from build123d import *

# Parameters (mm, degrees)
SKETCH2_W               = 42
SKETCH2_H               = 40
BOSS_EXTRUDE1_DEPTH     = 12.15
CUT_EXTRUDE1_DEPTH      = 149.231651478
CUT_EXTRUDE1_DEPTH_BACK = 149.231651478
SKETCH3_R               = 3.25
FILLET1_R               = 25
FILLET2_R               = 5
SKETCH4_R               = 3
BOSS_EXTRUDE2_DEPTH     = 2.8
CHAMFER1_SIZE           = 0.5
SKETCH6_W               = 20
SKETCH6_H               = 10.5
BOSS_EXTRUDE3_DEPTH     = 22
BOSS_EXTRUDE5_DEPTH     = 12
SKETCH7_R               = 1.65
CUT_EXTRUDE2_DEPTH      = 4
FILLET3_R               = 10
CHAMFER3_SIZE           = 2
SKETCH9_R               = 3.25
CUT_EXTRUDE3_DEPTH      = 2


# Some blends are built 0.0001 mm under size
with BuildPart() as part:
    # Sketch2 → Boss-Extrude1 (new, symmetric)
    with BuildSketch(Plane.XY):
        Polygon((-33, 0), (33, 0), (33, -144), (21, -144), (21, -99), (-21, -99), (-21, -144), (-33, -144), align=None)
        with Locations((0, -32)):
            Rectangle(SKETCH2_W, SKETCH2_H, mode=Mode.SUBTRACT)
        with Locations((0, -75.5)):
            Rectangle(SKETCH2_W, SKETCH2_H, mode=Mode.SUBTRACT)
    extrude(amount=BOSS_EXTRUDE1_DEPTH, both=True)

    # Sketch3 → Cut-Extrude1 (cut, two sides: drawn at the far end of the back side and taken through both)
    with BuildSketch(Plane(origin=(0, 0, 0), x_dir=(0, 0, -1), z_dir=(1, 0, 0)).offset(-CUT_EXTRUDE1_DEPTH_BACK)):
        with Locations((0, -106)):
            Circle(SKETCH3_R)
        with Locations((0, -62.5)):
            Circle(SKETCH3_R)
        with Locations((0, -19)):
            Circle(SKETCH3_R)
        with Locations((6, -134)):
            Circle(SKETCH3_R)
    extrude(amount=CUT_EXTRUDE1_DEPTH + CUT_EXTRUDE1_DEPTH_BACK, mode=Mode.SUBTRACT)

    # Fillet1
    # the kernel refuses this fillet: 25 mm, written as the material it takes off along each edge
    with BuildSketch(Plane(origin=(95.475495196, -144, 12.15), x_dir=(0, 1, 0), z_dir=(-1, 0, 0)), Plane(origin=(41.475495196, -144, 12.15), x_dir=(0, 1, 0), z_dir=(-1, 0, 0))) as fillet1_piece_1:
        with BuildLine():
            CenterArc((24.990198078, 25), FILLET1_R, 181.604491527, 88.395508473)
            Line((0, 24.3), (-0.499803962, 24.286))
            ThreePointArc((-0.499803962, 24.286), (-0.5, 12.15), (-0.5, 0))
            Line((-0.5, 0), (0, -0.5))
            Line((0, -0.5), (24.990198078, -0.5))
            Line((24.990198078, -0.5), (24.990198078, 0))
        make_face()
    extrude(amount=136.950990392, mode=Mode.SUBTRACT)

    # Fillet2
    fillet2_edges = [part.edges().sort_by_distance(p)[0] for p in [
        (-27, -144, -12.15),
        (27, -144, -12.15),
    ]]
    fillet(fillet2_edges, radius=FILLET2_R)

    # Sketch4 → Boss-Extrude2 (add)
    with BuildSketch(Plane(origin=(0, 0, 12.15), x_dir=(-1, 0, 0), z_dir=(0, 0, -1))):
        with Locations((-27, -6)):
            Circle(SKETCH4_R)
        with Locations((27, -6)):
            Circle(SKETCH4_R)
        with Locations((27, -106)):
            Circle(SKETCH4_R)
        with Locations((-27, -106)):
            Circle(SKETCH4_R)
    extrude(amount=-BOSS_EXTRUDE2_DEPTH)

    # Chamfer1
    chamfer1_edges = [part.edges().sort_by_distance(p)[0] for p in [
        (30, -6, 14.95),
        (-24, -6, 14.95),
        (-24, -106, 14.95),
        (30, -106, 14.95),
    ]]
    chamfer(chamfer1_edges, length=CHAMFER1_SIZE)

    # Sketch6 → Boss-Extrude3 (add)
    with BuildSketch(Plane(origin=(55, 0, 0), x_dir=(0, 0, -1), z_dir=(1, 0, 0))):
        with Locations((0, -26.14)):
            Rectangle(SKETCH6_W, SKETCH6_H)
        with Locations((0, -78.64)):
            Rectangle(SKETCH6_W, SKETCH6_H)
        Polygon((-0.922937771, -147.063882754), (18.427721371, -142.00898505), (21.081542665, -152.168081099), (1.730883524, -157.222978804), align=None)
        Polygon((-11.538222949, -95.575155055), (5.158614897, -91.213504805), (7.812436192, -101.372600854), (-11.538222949, -106.427498558), align=None)
    extrude(amount=-BOSS_EXTRUDE3_DEPTH)


with BuildPart() as boss_extrude3_piece_1:
    # of the separate pieces the step leaves, piece 1, a body of its own (boss_extrude3_pieces)
    add(part.part.solids().sort_by_distance((24, -106, 14.45))[0])



with BuildPart() as boss_extrude3_piece_2:
    # of the separate pieces the step leaves, piece 2, a body of its own (boss_extrude3_pieces)
    add(part.part.solids().sort_by_distance((55, -147.063882754, 0.922937771))[0])


with BuildPart() as boss_extrude3_piece_1_1:
    add(boss_extrude3_piece_1.part)

    add(boss_extrude3_piece_2.part)  # Boss-Extrude5 merges Boss-Extrude3 piece 2
    # Sketch8 → Boss-Extrude5 (add)
    with BuildSketch(Plane(origin=(33, 0, 0), x_dir=(0, 0, -1), z_dir=(1, 0, 0))):
        with BuildLine():
            Line((-0.922937771, -147.063882754), (-3.256769685, -138.129738384))
            ThreePointArc((-3.256769685, -138.129738384), (0.984375203, -141.014504786), (5.725, -142.972989836))
            ThreePointArc((5.725, -142.972989836), (10.139565186, -142.188157138), (12.15, -138.180352253))
            Line((12.15, -138.180352253), (12.15, -117.977233364))
            Line((12.15, -117.977233364), (18.427721371, -142.00898505))
            Line((18.427721371, -142.00898505), (21.081542665, -152.168081099))
            Line((21.081542665, -152.168081099), (1.730883524, -157.222978804))
            Line((1.730883524, -157.222978804), (-0.922937771, -147.063882754))
        make_face()
    extrude(amount=-BOSS_EXTRUDE5_DEPTH)

    # Sketch7 → Cut-Extrude2 (cut)
    with BuildSketch(Plane(origin=(55, 0, 0), x_dir=(0, 0, -1), z_dir=(1, 0, 0))):
        with Locations((-4.75, -27.89)):
            Circle(SKETCH7_R)
        with Locations((4.75, -27.89)):
            Circle(SKETCH7_R)
        with Locations((-4.75, -76.89)):
            Circle(SKETCH7_R)
        with Locations((4.75, -76.89)):
            Circle(SKETCH7_R)
        with Locations((-7.343282023, -101.714222561)):
            Circle(SKETCH7_R)
        with Locations((1.848281069, -99.313146151)):
            Circle(SKETCH7_R)
        with Locations((5.041217352, -149.123337457)):
            Circle(SKETCH7_R)
        with Locations((14.232780444, -146.722261047)):
            Circle(SKETCH7_R)
    extrude(amount=-CUT_EXTRUDE2_DEPTH, mode=Mode.SUBTRACT)

    # Fillet3
    fillet3_edges = [boss_extrude3_piece_1_1.edges().sort_by_distance(p)[0] for p in [
        (38, -157.222978804, -1.730883524),
        (38, -152.168081099, -21.081542665),
        (27, -117.977233364, -12.15),
        (27, -138.129738384, 3.256769685),
    ]]
    fillet(fillet3_edges, radius=FILLET3_R - 0.0001)  # a hair under: the kernel refuses the full size

    # Chamfer3
    # the kernel refuses this chamfer: 2 mm, written as the material it adds along each edge
    with BuildSketch(Plane(origin=(33, -20.89, 2.499429517), x_dir=(-0.027495876610585647, 0.9996219169112968, 0), z_dir=(0, 0, -1))) as chamfer3_piece_1_section:
        Polygon((CHAMFER3_SIZE * 0.999621916911, CHAMFER3_SIZE * 0.0274958766106), (-CHAMFER3_SIZE * 0.0274958766106, CHAMFER3_SIZE * 0.999621916911), (0, 0), align=None)
    chamfer3_piece_1 = extrude(amount=12.499429517, mode=Mode.PRIVATE)
    chamfer3_piece_1 = chamfer3_piece_1 - Plane(origin=(33.672455273, -19, 0), x_dir=(0, 0, -1), z_dir=(-1, 0, 0)) * Cylinder(3.25, 33, mode=Mode.PRIVATE)
    add(chamfer3_piece_1)
    with BuildSketch(Plane(origin=(33, -20.89, 10), x_dir=(-0.027495876610585647, 0.9996219169112968, 0), z_dir=(0, 0, -1))) as chamfer3_piece_2_section:
        Polygon((CHAMFER3_SIZE * 0.999621916911, CHAMFER3_SIZE * 0.0274958766106), (-CHAMFER3_SIZE * 0.0274958766106, CHAMFER3_SIZE * 0.999621916911), (0, 0), align=None)
    chamfer3_piece_2 = extrude(amount=12.499429517, mode=Mode.PRIVATE)
    chamfer3_piece_2 = chamfer3_piece_2 - Plane(origin=(33.672455268, -19, 0), x_dir=(0, 0, -1), z_dir=(-1, 0, 0)) * Cylinder(3.25, 33, mode=Mode.PRIVATE)
    add(chamfer3_piece_2)
    with BuildSketch(Plane(origin=(33, -31.39, -10), x_dir=(-0.027495876610585647, -0.9996219169112968, 0), z_dir=(0, 0, 1)), Plane(origin=(33, -73.39, 10), x_dir=(-0.02749587661058555, 0.9996219169112968, 0), z_dir=(0, 0, -1)), Plane(origin=(33, -83.89, -10), x_dir=(-0.02749587661058555, -0.9996219169112968, 0), z_dir=(0, 0, 1)), Plane(origin=(33, -147.063882754, 0.922937771), x_dir=(-0.02749587661058553, 0.9671671492128019, 0.25264932664267514), z_dir=(0, 0.2527448852095291, -0.96753295706163))) as chamfer3_piece_3:
        Polygon((CHAMFER3_SIZE * 0.999621916911, CHAMFER3_SIZE * 0.0274958766106), (-CHAMFER3_SIZE * 0.0274958766106, CHAMFER3_SIZE * 0.999621916911), (0, 0), align=None)
    extrude(amount=20)
    with BuildSketch(Plane(origin=(33, -102.802754601, -2.337663147), x_dir=(-0.027495876610585706, -0.9671671492128018, -0.25264932664267636), z_dir=(0, -0.2527448852095303, 0.9675329570616298))) as chamfer3_piece_4_section:
        Polygon((CHAMFER3_SIZE * 0.999621916911, CHAMFER3_SIZE * 0.0274958766106), (-CHAMFER3_SIZE * 0.0274958766106, CHAMFER3_SIZE * 0.999621916911), (0, 0), align=None)
    chamfer3_piece_4 = extrude(amount=19.484878578, mode=Mode.PRIVATE)
    chamfer3_piece_4 = chamfer3_piece_4 - Plane(origin=(33.819409297, -106, 0), x_dir=(0, 0, -1), z_dir=(-1, 0, 0)) * Cylinder(3.25, 47, mode=Mode.PRIVATE)
    chamfer3_piece_4 = split(chamfer3_piece_4, bisect_by=Plane(origin=(33.819409297, -103.234814786, 11.538222949), z_dir=(0, 0, -1)), keep=Keep.TOP, mode=Mode.PRIVATE)
    add(chamfer3_piece_4)
    with BuildSketch(Plane(origin=(33, -96.875114499, 16.514599041), x_dir=(-0.027495876610585716, 0.967167149212802, 0.2526493266426752), z_dir=(0, 0.2527448852095292, -0.96753295706163))) as chamfer3_piece_5_section:
        Polygon((CHAMFER3_SIZE * 0.999621916911, CHAMFER3_SIZE * 0.0274958766106), (-CHAMFER3_SIZE * 0.0274958766106, CHAMFER3_SIZE * 0.999621916911), (0, 0), align=None)
    chamfer3_piece_5 = extrude(amount=22.400491663, mode=Mode.PRIVATE)
    chamfer3_piece_5 = split(chamfer3_piece_5, bisect_by=Plane(origin=(33.668365734, -92.730700089, 11.538222949), z_dir=(0, 0, -1)), keep=Keep.TOP, mode=Mode.PRIVATE)
    add(chamfer3_piece_5)
    with BuildSketch(Plane(origin=(33, -101.372600854, -7.812436192), x_dir=(-0.027495876610585706, -0.9671671492128017, -0.25264932664267636), z_dir=(0, -0.2527448852095303, 0.9675329570616298))) as chamfer3_piece_6_section:
        Polygon((CHAMFER3_SIZE * 0.999621916911, CHAMFER3_SIZE * 0.0274958766106), (-CHAMFER3_SIZE * 0.0274958766106, CHAMFER3_SIZE * 0.999621916911), (0, 0), align=None)
    chamfer3_piece_6 = extrude(amount=11.798194515, mode=Mode.PRIVATE)
    chamfer3_piece_6 = chamfer3_piece_6 - Plane(origin=(33.67836444, -106, 0), x_dir=(0, 0, -1), z_dir=(-1, 0, 0)) * Cylinder(3.25, 32, mode=Mode.PRIVATE)
    add(chamfer3_piece_6)

    # Sketch9 → Cut-Extrude3 (cut)
    with BuildSketch(Plane(origin=(33, 0, 0), x_dir=(0, 0, -1), z_dir=(1, 0, 0))):
        with Locations((0, -19)):
            Circle(SKETCH9_R)
        with Locations((0, -106)):
            Circle(SKETCH9_R)
    extrude(amount=CUT_EXTRUDE3_DEPTH, mode=Mode.SUBTRACT)


solid = boss_extrude3_piece_1_1.part
Part model, mm, in its own coordinate system. A direction names the side the tool comes from. Round coordinates to 2 decimals unless told otherwise and drop trailing zeros. Write each loop counter-clockwise with the first axis right and the second up, starting at its lowest first coordinate (ties: lowest second). Pieces come first, ordered by that corner, then holes. Notation, with made-up numbers: (15.25, -39) - (52.25, -39) arc R14 ccw to (52.25, -33) - close; hole circle Ø4 at (44.5, -24). An arc over 180 degrees is marked (long way). Use CSV: the item, a comma, the result in double quotes.
Item 1: Flat gauge pins, fed straight in: P1, Ø1.5, axis at x = -16.5, z = -5.5, coming from the -Y side; P2, Ø1.7, axis at y = -102, z = 7, coming from the +X side; P3, Ø1.5, axis at y = -55.5, z = -4.5, coming from the +X side. Where does each tip first touch, or does it go through?
Results list:
P1,"stops at y = -99"
P2,"stops at x = 51"
P3,"stops at x = 33"
Item 2: Wall check: L1, parallel to Y at x = -11, z = -5.5; L2, parallel to X at y = -77, z = 0.5; L3, parallel to Y at x = 52.1, z = 4.75. Give the ranges that are in metal, low to high.
Results list:
L1,"y = -99 to -95.5, -55.5 to -52, -12 to 0"
L2,"x = -33 to -21, 21 to 55"
L3,"y = -104.65 to -93.8, -83.89 to -78.54, -75.24 to -73.39, -31.39 to -29.54, -26.24 to -20.89"
Item 3: Pull direction Y, two halves, no side cores. Call faces 1 (the cylindrical face through (26.92, -138.56, 3.48)), 2 (the cylindrical face through (53.028, -103.325, 7.701)), 3 (the flat face through (44, -26, -10)): pulls with the +Y half, pulls with the -Y half, needs draft (parallel to the pull), parting line crosses it, or undercut.
Results list:
face 1,"pulls with the -Y half"
face 2,"undercut"
face 3,"needs draft"
Item 4: Tool access for faces 4 (the cylindrical face through (-26.35, -108.93, 13.28)), 5 (the cylindrical face through (53.03, -150.59, -5.8)), 6 (the flat face through (33.99, -103.18, -4.89)), 7 (the flat face through (44, -79, 10)), 8 (the flat face through (0, -99, 0)): list every direction of +Z, -Z, +X, -X, +Y, -Y with a clear straight run to the whole face (end or side of a thin tool).
Results list:
face 4,"+Z"
face 5,"+X"
face 6,"-Z, +X"
face 7,"+Z, +X, +Y"
face 8,"+Z, -Z, -Y"
Item 5: Slice it at D-D, the plane x = 37. Count the separate pieces of the cut face and the enclosed holes in it, then the cut area to 3 significant figures.
Results list:
separate pieces,"4"
enclosed holes,"0"
area,"783 mm²"
Item 6: Slice it at A-A, the plane y = -44. Write the cut outline in (x, z), then the cut area to 3 significant figures.
Results list:
outline,"(-33, -12.15) - (-21, -12.15) - (-21, 12.15) - (-33, 12.15) - close; (21, -12.15) - (33, -12.15) - (33, 12.15) - (21, 12.15) - close"
area,"583 mm²"
Item 7: Slice it at C-C, the plane x = -27. Write the cut outline in (y, z) (3 decimals), then the cut area to 3 significant figures.
Results list:
outline,"(-142.973, -5.725) arc R5 ccw to (-138.18, -12.15) - (0, -12.15) - (0, 12.15) - (-3, 12.15) - (-3, 14.45) - (-3.5, 14.95) - (-8.5, 14.95) - (-9, 14.45) - (-9, 12.15) - (-103, 12.15) - (-103, 14.45) - (-103.5, 14.95) - (-108.5, 14.95) - (-109, 14.45) - (-109, 12.15) - (-119.01, 12.15) arc R25 ccw to start; hole circle Ø6.5 at (-134, -6); hole circle Ø6.5 at (-106, 0); hole circle Ø6.5 at (-62.5, 0); hole circle Ø6.5 at (-19, 0)"
area,"3,260 mm²"
Item 8: Slice it at B-B, the plane x = -11.5. Write the cut outline in (y, z).
Results list:
outline,"(-99, -12.15) - (-95.5, -12.15) - (-95.5, 12.15) - (-99, 12.15) - close; (-55.5, -12.15) - (-52, -12.15) - (-52, 12.15) - (-55.5, 12.15) - close; (-12, -12.15) - (0, -12.15) - (0, 12.15) - (-12, 12.15) - close"
